from build123d import *

# Parameters (mm, degrees)
F1_DEPTH = 5


# Not quite as in the source:
# - a feature names something its author has since deleted; it is built from what else it names


with BuildPart() as f1:
    # F0 (on Top) → F1 (new body)
    with BuildSketch(Plane.XY):
        with BuildLine():
            Line((0, -16), (0, -120))
            ThreePointArc((0, -120), (120, 0), (0, 120))
            Line((0, 120), (0, 16))
            ThreePointArc((0, 16), (11.313708499, 11.313708499), (16, 0))
            ThreePointArc((16, 0), (11.313708499, -11.313708499), (0, -16))
        make_face()
    extrude(amount=F1_DEPTH)


solid = f1.part
Design review of the part built by this model. Coordinates are the model's own, in mm. Give positions to 0.01 mm unless a question says otherwise; leave off trailing zeros. Order: outer loops, then holes, each group sorted by start corner. A loop starts at its lowest first (then second) coordinate and runs counter-clockwise, first axis right, second up. Notation, with made-up numbers: (59, 62.5) - (79, 62.5) arc R24 ccw to (79, 73.5) - close; hole circle Ø6 at (19.5, -17.75). An arc over 180 degrees is marked (long way). Use CSV: the item, a comma, the result in double quotes. Start each with the question number.
Q1. Take a section at A-A (x = 13.5). State the section outline as (y, z) points.
Q2. Take a section at B-B (z = 3.5). State the section outline as (x, y) points.
Q3. For line 1 (Y direction, x = 10.5, z = 1.2); line 2 (Y direction, x = 67, z = 4.05); line 3 (X direction, y = 51.5, z = 3.9), list the stretches that pass through material, from the lowest coordinate up.
Q4. Take a section at D-D (x = 38). State the section outline as (y, z) points, and give its area (3 significant figures).
Q5. Take a section at C-C (y = -85.5). State the section outline as (x, z) points.
Q6. For P1, Ø2, axis at x = 73.5, z = 4.5, coming from the +Y side; P2, Ø3, axis at x = 80, z = 0.5, coming from the -Y side; P3, Ø1.5, axis at x = 33.5, z = 2.5, coming from the +Y side; P4, Ø4, axis at x = 36, y = -35.5, coming from the -Z side, all flat-tipped, find the tip position at first contact; note any pin that passes through.
Calculated:
1,outline,"(-119.24, 0) - (-8.59, 0) - (-8.59, 5) - (-119.24, 5) - close; (8.59, 0) - (119.24, 0) - (119.24, 5) - (8.59, 5) - close"
2,outline,"(0, -120) arc R120 ccw to (0, 120) - (0, 16) arc R16 cw to (0, -16) - close"
3,line 1,"y = -119.54 to -12.07, 12.07 to 119.54"
3,line 2,"y = -99.55 to 99.55"
3,line 3,"x = 0 to 108.39"
4,outline,"(-113.82, 0) - (113.82, 0) - (113.82, 5) - (-113.82, 5) - close"
4,area,"1,140 mm²"
5,outline,"(0, 0) - (84.2, 0) - (84.2, 5) - (0, 5) - close"
6,P1,"stops at y = 95.62"
6,P2,"stops at y = -90.76"
6,P3,"stops at y = 115.44"
6,P4,"stops at z = 0"
